Design review of the part shown in the three views and the two pictorial views. Dimensions are in mm from the part's minimum x, y and z. Coordinates: 2 decimals unless noted, no trailing zeros. Loops run counter-clockwise (first coordinate to the right, second up) from the corner with the lowest first, then second, coordinate; pieces in that order, holes last. Notation, with made-up numbers: M -21.75,39 L 33.25,39 A9 cw 33.25,49 Z; hole C -19.5,65.5 d7. An arc over 180 degrees is marked long. Use one line per item in the form item = value.
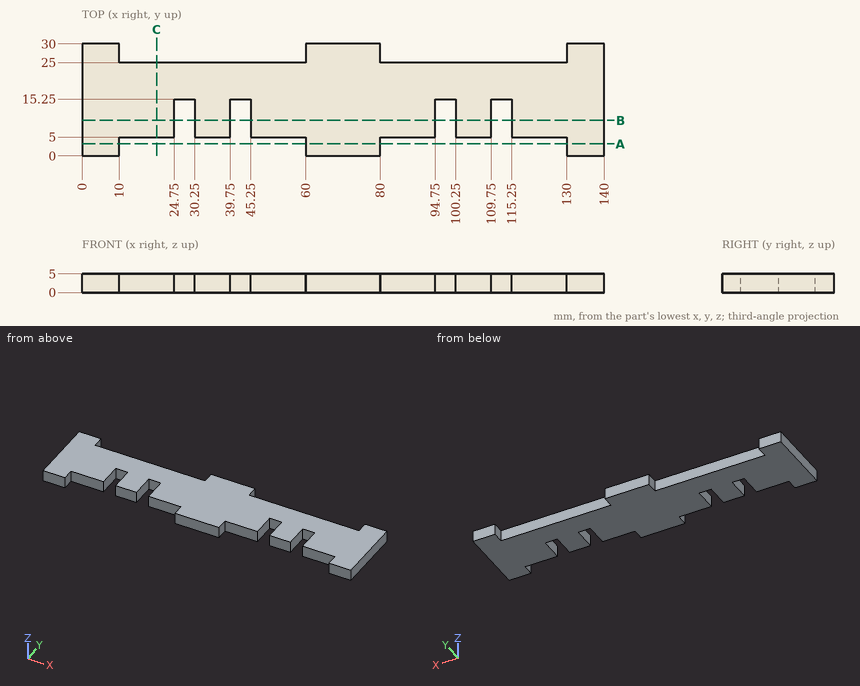
1. Add section B-B (y = 9.5). State the section outline as (x, z) points, then the cut area to 3 significant figures.
Response values:
outline = M 0,0 L 24.75,0 L 24.75,5 L 0,5 Z; M 30.25,0 L 39.75,0 L 39.75,5 L 30.25,5 Z; M 45.25,0 L 94.75,0 L 94.75,5 L 45.25,5 Z; M 100.25,0 L 109.75,0 L 109.75,5 L 100.25,5 Z; M 115.25,0 L 140,0 L 140,5 L 115.25,5 Z
area = 590 mm^2
2. Add section A-A (y = 3.25). State the section outline as (x, z) points, then the cut area to 3 significant figures.
Response values:
outline = M 0,0 L 10,0 L 10,5 L 0,5 Z; M 60,0 L 80,0 L 80,5 L 60,5 Z; M 130,0 L 140,0 L 140,5 L 130,5 Z
area = 200 mm^2
3. Add section C-C (x = 20). State the section outline as (y, z) points.
Response values:
outline = M 5,0 L 25,0 L 25,5 L 5,5 Z
4. Insertion check: P1, Ø2.5, axis at x = 27, z = 3.5, coming from the -Y side; P2, Ø2.5, axis at x = 106, z = 2.5, coming from the -Y side. Each pin has a flat end and moves straight along its axis. Give the tip position at first contact, or say it passes through.
Response values:
P1 = 15.25
P2 = 5
5. Wall thickness on line 1 along X through (y, z) = (10.5, 3); line 2 along X through (y, z) = (27.75, 2.8); line 3 along Y through (x, z) = (119.5, 1.35): over which ranges is each line inside the solid? List them lowest first. Write a range as from..to.
Response values:
line_1 = 0..24.75, 30.25..39.75, 45.25..94.75, 100.25..109.75, 115.25..140
line_2 = 0..10, 60..80, 130..140
line_3 = 5..25
